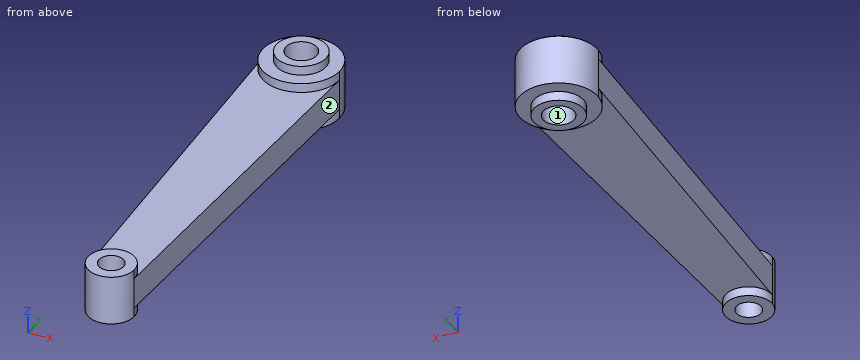
Autodesk Inventor part; units mm, degrees
ref_plane "YZ Plane" through (0, 0, 0) normal (1, 0, 0) x (0, 1, 0)
ref_plane "XZ Plane" through (0, 0, 0) normal (0, 1, 0) x (-1, 0, 0)
ref_plane "XY Plane" through (0, 0, 0) normal (0, 0, 1) x (1, 0, 0)
sketch "Sketch1" plane through (0, 0, 0) normal (0, 0, 1) x (1, 0, 0)
  line L0 (-17.5, 0) -> (17.5, 0)
  line L1 (0, -95.0833) -> (0, 100.9167)
  arc A0 (12.4891, 59.8958) -> (-12.4891, 59.8958) centre (0, 60.4167) ccw
  arc A1 (-7.4935, -59.8958) -> (7.4935, -59.8958) centre (0, -59.5833) ccw
  line L2 (-12.4891, 59.8958) -> (-7.4935, -59.8958)
  line L3 (12.4891, 59.8958) -> (7.4935, -59.8958)
  point P0 (0, 0)
  point P1 (-9.9913, 0)
  dimension "d0" = 25
  dimension "d1" = 15
  dimension "d2" = 120
extrude "Extrusion1" add sketch "Sketch1" along normal mid plane 10
sketch "Sketch2" plane through (0, 0, 0) normal (0, 0, 1) x (1, 0, 0)
  line L0 (-7.4935, -59.8958) -> (-12.4891, 59.8958)
  arc A0 (12.4891, 59.8958) -> (-12.4891, 59.8958) centre (0, 60.4167) ccw
  line L1 (12.4891, 59.8958) -> (7.4935, -59.8958)
  arc A1 (-7.4935, -59.8958) -> (7.4935, -59.8958) centre (0, -59.5833) ccw
  circle A2 centre (0, 60.4167) radius 12.5
  circle A3 centre (0, -59.5833) radius 7.5
  point P0 (0, 0)
extrude "Extrusion2" add sketch "Sketch2" along normal mid plane 16 contours A3 A1 | A0 A2
sketch "Sketch3" plane through (0, 0, 0) normal (0, 0, 1) x (1, 0, 0)
  circle A0 centre (0, 60.4167) radius 8
  circle A1 centre (0, 60.4167) radius 12.5
  point P0 (0, 0)
  dimension "d7" = 16
extrude "Extrusion3" add sketch "Sketch3" along normal mid plane 22 contours A0
sketch "Sketch4" plane through (0, 0, 0) normal (0, 0, 1) x (1, 0, 0)
  arc A0 (7.4935, -59.8958) -> (-7.4935, -59.8958) centre (0, -59.5833) ccw
  line L0 (-7.4935, -59.8958) -> (-12.4891, 59.8958)
  arc A1 (-12.4891, 59.8958) -> (12.4891, 59.8958) centre (0, 60.4167) ccw
  line L1 (12.4891, 59.8958) -> (7.4935, -59.8958)
  circle A2 centre (0, 60.4167) radius 8
  circle A3 centre (0, 60.4167) radius 12.5
  circle A4 centre (0, -59.5833) radius 7.5
  circle A5 centre (0, 60.4167) radius 5
  circle A6 centre (0, -59.5833) radius 4
  point P0 (0, 0)
  dimension "d10" = 10
  dimension "d11" = 8
extrude "Extrusion4" cut sketch "Sketch4" along normal through all both and the other way through all contours A5 | A6
properties part number "Connector_Rod" material "Steel, Carbon"
Work out the finished part from the listing and answer in its coordinate system (mm). Face numbers are marked on the shaded views. Coordinates: 2 decimals unless noted, no trailing zeros. Order: outer loops, then holes, each group sorted by start corner. A loop starts at its lowest first (then second) coordinate and runs counter-clockwise, first axis right, second up. Notation, with made-up numbers: (25, 42.5) - (38, 42.5) arc R32 ccw to (38, 74.5) - close; hole circle Ø1 at (-26.75, -18.5). An arc over 180 degrees is marked (long way). Put each result on its own line as item: value. Start each with the question number.
1) Find section D-D (y = 22). Give the vertices of the cut face in (x, z).
2) Find the intervals of material crossed by line 1 (Y direction, x = 0, z = 1.5); line 2 (Z direction, x = -6.25, y = -40); line 3 (Y direction, x = -2.5, z = 1), in increasing order. Write a range as from..to.
3) For a pull along Y with two mould halves and no side action, classify the marked faces 1 and 2 as released by +Y, released by -Y, zero draft, split by the parting line, or undercut.
4) Flat-ended cylindrical pins translate along their axes: pin 1 (1.5 mm diameter, centred on x = -5.5, z = 4.5, fed in from +Y); pin 2 (10 mm diameter, centred on x = -7, y = -13.5, fed in from +Z); pin 3 (12 mm diameter, centred on y = -31.5, z = 8.5, fed in from -X); pin 4 (8 mm diameter, centred on x = -1, z = 6.5, fed in from +Y). Find the tip coordinate at first contact, or state that the pin passes through.
5) Find section C-C (x = 10). Give the vertices of the cut face in (y, z), plus the area to 3 significant figures.
6) Find section B-B (z = 1). Give the vertices of the cut face in (x, y).
7) Find section A-A (x = 0). Give the vertices of the cut face in (y, z).
Results list:
1. outline: (-10.91, -5) - (10.91, -5) - (10.91, 5) - (-10.91, 5) - close
2. line 1: y = -67.08..-63.58, -55.58..55.42, 65.42..72.92
2. line 2: z = -5..5
2. line 3: y = -66.65..-62.71, -56.46..56.09, 64.75..72.66
3. face 1: undercut
3. face 2: released by -Y
4. pin 1: stops at y = 71.98
4. pin 2: stops at z = 5
4. pin 3: stops at x = -8.88
4. pin 4: stops at y = 72.92
5. outline: (0.21, -5) - (52.92, -5) - (52.92, -8) - (67.92, -8) - (67.92, 8) - (52.92, 8) - (52.92, 5) - (0.21, 5) - close
5. area: 767 mm^2
6. outline: (-12.49, 59.9) - (-7.49, -59.9) arc R7.5 ccw to (7.49, -59.9) - (12.49, 59.9) arc R12.5 ccw (long way) to start; hole circle Ø10 at (0, 60.42); hole circle Ø8 at (0, -59.58)
7. outline: (-67.08, -8) - (-63.58, -8) - (-63.58, 8) - (-67.08, 8) - close; (-55.58, -8) - (-52.08, -8) - (-52.08, -5) - (47.92, -5) - (47.92, -8) - (52.42, -8) - (52.42, -11) - (55.42, -11) - (55.42, 11) - (52.42, 11) - (52.42, 8) - (47.92, 8) - (47.92, 5) - (-52.08, 5) - (-52.08, 8) - (-55.58, 8) - close; (65.42, -11) - (68.42, -11) - (68.42, -8) - (72.92, -8) - (72.92, 8) - (68.42, 8) - (68.42, 11) - (65.42, 11) - close
